Work out the finished part from the listing and answer in its coordinate system (mm). Face numbers are marked on the shaded views. A direction names the side the tool comes from. Coordinates: 2 decimals unless noted, no trailing zeros. Loops run counter-clockwise (first coordinate to the right, second up) from the corner with the lowest first, then second, coordinate; pieces in that order, holes last.
```python
from build123d import *

# Parameters (mm, degrees)
SALIENTE_EXTRUIR1_DEPTH = 5
CROQUIS2_W              = 16
CROQUIS2_H              = 5
SALIENTE_EXTRUIR2_DEPTH = 10
CORTAR_EXTRUIR1_REACH   = 7
CROQUIS3_R              = 2


with BuildPart() as part:
    # Croquis1 → Saliente-Extruir1 (new body)
    with BuildSketch(Plane.XY):
        Polygon((-110, 25), (-73, 25), (-73, 0), (-57, 0), (-57, 25), (57, 25), (57, 0), (73, 0), (73, 25), (110, 25), (110, 35), (-110, 35), align=None)
    extrude(amount=SALIENTE_EXTRUIR1_DEPTH)

    # Croquis2 → Saliente-Extruir2 (add)
    with BuildSketch(Plane(origin=(0, 0, 0), x_dir=(-1, 0, 0), z_dir=(0, 0, -1))):
        with Locations((65, 2.5)):
            Rectangle(CROQUIS2_W, CROQUIS2_H)
        with Locations((-65, 2.5)):
            Rectangle(CROQUIS2_W, CROQUIS2_H)
    extrude(amount=SALIENTE_EXTRUIR2_DEPTH)

    # Croquis3 → Cortar-Extruir1 (cut, up to next)
    with BuildSketch(Plane(origin=(0, 5, 0), x_dir=(1, 0, 0), z_dir=(0, 1, 0)), mode=Mode.PRIVATE) as cortar_extruir1_sk1:
        with Locations((65, 5)):
            Circle(CROQUIS3_R)
    cortar_extruir1_tool1 = extrude(cortar_extruir1_sk1.sketch, amount=-CORTAR_EXTRUIR1_REACH, mode=Mode.PRIVATE) & part.part
    add(cortar_extruir1_tool1.solids().sort_by_distance((65, 5, -5))[0], mode=Mode.SUBTRACT)
    # Croquis3 → Cortar-Extruir1 (cut, up to next)
    with BuildSketch(Plane(origin=(0, 5, 0), x_dir=(1, 0, 0), z_dir=(0, 1, 0)), mode=Mode.PRIVATE) as cortar_extruir1_sk2:
        with Locations((-65, 5)):
            Circle(CROQUIS3_R)
    cortar_extruir1_tool2 = extrude(cortar_extruir1_sk2.sketch, amount=-CORTAR_EXTRUIR1_REACH, mode=Mode.PRIVATE) & part.part
    add(cortar_extruir1_tool2.solids().sort_by_distance((-65, 5, -5))[0], mode=Mode.SUBTRACT)


solid = part.part
```
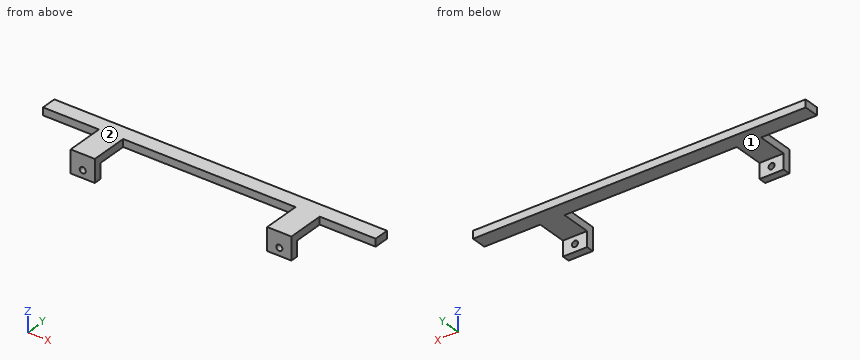
1. Straight lines are drawn through the part: probe 1 along X at (y, z) = (1.8, -5); probe 2 along Z at (x, y) = (-65, 1.35); probe 3 along X at (y, z) = (20.5, 3.75). For each, find the intervals that lie inside material, in ascending order.
2. A cutting plane is placed at C-C, the plane z = -5. Give the vertices of the cut face in (x, y), then the cut area to 3 significant figures.
3. A cutting plane is placed at B-B, the plane y = 8.5. Give the vertices of the cut face in (x, z).
4. For the marked faces 1 and 2, determine the directions among +Z, -Z, +X, -X, +Y, -Y from which every point of the face is accessible in a straight line to the end or side of a thin tool.
5. A cutting plane is placed at D-D, the plane y = 29. Give the vertices of the cut face in (x, z), then the cut area to 3 significant figures.
6. A cutting plane is placed at A-A, the plane x = 65. Give the vertices of the cut face in (y, z).
7. Each of these flat-tipped pins is pushed along its axis until it touches: P1, Ø4.5, axis at y = 7, z = -3, coming from the -X side; P2, Ø8, axis at x = -5.5, z = -1, coming from the -Y side; P3, Ø8, axis at x = -61, z = -6, coming from the +Y side. Where does it stop, or does it pass through?
Answers below:
1. probe 1: x = -73 to -67, -63 to -57, 57 to 63, 67 to 73
1. probe 2: z = -10 to -7, -3 to 5
1. probe 3: x = -73 to -57, 57 to 73
2. outline: (-73, 0) - (-67, 0) - (-67, 5) - (-73, 5) - close; (-63, 0) - (-57, 0) - (-57, 5) - (-63, 5) - close; (57, 0) - (63, 0) - (63, 5) - (57, 5) - close; (67, 0) - (73, 0) - (73, 5) - (67, 5) - close
2. area: 120 mm2
3. outline: (-73, 0) - (-57, 0) - (-57, 5) - (-73, 5) - close; (57, 0) - (73, 0) - (73, 5) - (57, 5) - close
4. face 1: -Z, +X, -X, +Y
4. face 2: +Z, +X, -X, +Y, -Y
5. outline: (-110, 0) - (110, 0) - (110, 5) - (-110, 5) - close
5. area: 1,100 mm2
6. outline: (0, -10) - (5, -10) - (5, -7) - (0, -7) - close; (0, -3) - (5, -3) - (5, 0) - (35, 0) - (35, 5) - (0, 5) - close
7. P1: stops at x = -73
7. P2: stops at y = 25
7. P3: stops at y = 5
